The model under review builds one solid part; all positions refer to its coordinate system, in mm. Coordinates: 2 decimals unless noted, no trailing zeros. Loops run counter-clockwise (first coordinate to the right, second up) from the corner with the lowest first, then second, coordinate; pieces in that order, holes last. Notation, with made-up numbers: M 78.25,82.5 L 103.25,82.5 A14 ccw 103.25,93.5 Z; hole C 54.25,60.5 d3. An arc over 180 degrees is marked long. Use CSV: the item, a comma, the result in double quotes. Start each with the question number.
1. For L1, parallel to X at y = 947, z = 26; L2, parallel to Z at x = 28.5, y = 1266.5; L3, parallel to Z at x = -33, y = 1471.5, list the stretches that pass through material, from the lowest coordinate up.
2. Add section B-B, the plane y = 739. Write out the cut boundary in (x, z), then the cut area to 3 significant figures.
3. Add section A-A, the plane z = 16.5. Write out the cut boundary in (x, y).
4. Clearance check with flat-ended pins moving along their axes: P1, Ø8, axis at x = -29.5, y = 201, coming from the +Z side; P2, Ø2, axis at x = 13.5, y = 1636.5, coming from the +Z side. State where each tip first meets the part, or that it passes through.
5. Add section C-C, the plane x = 11. Write out the cut boundary in (y, z).
from build123d import *

# Parameters (mm, degrees)
C_CHANNEL_80_X_8_1_DEPTH = 1900


with BuildPart() as part:
    # Sketch11 → C channel 80 X 8(1) (new body)
    with BuildSketch(Plane.ZX):
        with BuildLine():
            Line((0, -37.5), (0, 37.5))
            Line((0, 37.5), (40, 37.5))
            Line((40, 37.5), (40, 34.5))
            ThreePointArc((40, 34.5), (38.535533906, 30.964466094), (35, 29.5))
            Line((35, 29.5), (8, 29.5))
            Line((8, 29.5), (8, -29.5))
            Line((8, -29.5), (35, -29.5))
            ThreePointArc((35, -29.5), (38.535533906, -30.964466094), (40, -34.5))
            Line((40, -34.5), (40, -37.5))
            Line((40, -37.5), (0, -37.5))
        make_face()
    extrude(amount=C_CHANNEL_80_X_8_1_DEPTH)


solid = part.part
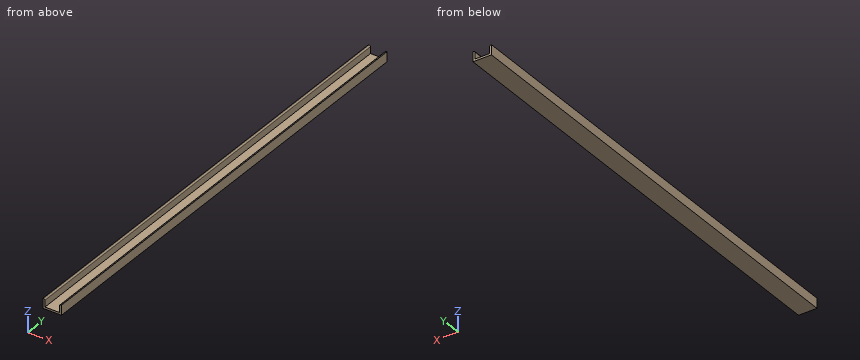
Computed:
1,L1,"x = -37.5 to -29.5, 29.5 to 37.5"
1,L2,"z = 0 to 8"
1,L3,"z = 0 to 39.77"
2,outline,"M -37.5,0 L 37.5,0 L 37.5,40 L 34.5,40 A5 ccw 29.5,35 L 29.5,8 L -29.5,8 L -29.5,35 A5 ccw -34.5,40 L -37.5,40 Z"
2,area,"1,100 mm^2"
3,outline,"M -37.5,0 L -29.5,0 L -29.5,1900 L -37.5,1900 Z; M 29.5,0 L 37.5,0 L 37.5,1900 L 29.5,1900 Z"
4,P1,"stops at z = 39.9"
4,P2,"stops at z = 8"
5,outline,"M 0,0 L 1900,0 L 1900,8 L 0,8 Z"
